Read the model definition and answer for the solid it produces. Units are mm, in the model's axes. Coordinates: 2 decimals unless noted, no trailing zeros. Loops run counter-clockwise (first coordinate to the right, second up) from the corner with the lowest first, then second, coordinate; pieces in that order, holes last. Notation, with made-up numbers: M 67.25,47 L 87.25,47 A10 ccw 87.25,60 Z; hole C 24.25,-1 d11. An arc over 180 degrees is marked long. One line per item, written item: value. Start each with the question number.
1. The part is cut by section B-B (x = 136.5). Write down the section's boundary in (y, z), then the cut area to 3 significant figures.
2. Consider probe 1 along Z at (x, y) = (167, -39.5). Determine where the line is inside the solid, lowest interval first.
3. The part is cut by section A-A (z = -138.5). Write down the section's boundary in (x, y), then the cut area to 3 significant figures.
4. The part is cut by section C-C (y = 100). Write down the section's boundary in (x, z).
5. Flat-ended cylindrical pins translate along their axes: pin 1 (6.5 mm diameter, centred on x = -4, z = -214.5, fed in from -Y); pin 2 (5.5 mm diameter, centred on x = 124.5, z = 2, fed in from -Y); pin 3 (5 mm diameter, centred on x = 287.5, z = -217, fed in from -Y). Find the tip coordinate at first contact, or state that the pin passes through.
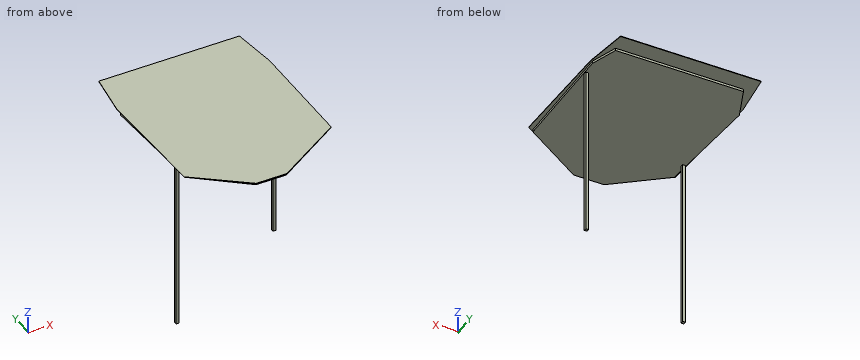
```python
from build123d import *

# Parameters (mm, degrees)
ESQUISSE1_W        = 50
ESQUISSE1_H        = 50
BOSS_EXTRU_1_DEPTH = 5
BOSS_EXTRU_2_DEPTH = 5
ESQUISSE3_W        = 6
ESQUISSE3_H        = 6
BOSS_EXTRU_3_DEPTH = 350
BOSS_EXTRU_4_DEPTH = 1


with BuildPart() as part:
    # Esquisse1 → Boss.-Extru.1 (new body)
    with BuildSketch(Plane.XY):
        with Locations((25, 25)):
            Rectangle(ESQUISSE1_W, ESQUISSE1_H)
    extrude(amount=BOSS_EXTRU_1_DEPTH)

    # Esquisse2 → Boss.-Extru.2 (add)
    with BuildSketch(Plane.XY.offset(5)):
        Polygon((-17.13807747, 66.750016637), (11.246380261, 134.000915956), (274.564409595, 134.000915956), (292.219085418, 78.963245992), (285.658191139, -157.093376415), (157.625700404, -238.014344585), (94.995088054, -238.014344585), (-5.374322013, -157.093376415), align=None)
    extrude(amount=-BOSS_EXTRU_2_DEPTH)

    # Esquisse3 → Boss.-Extru.3 (add)
    with BuildSketch(Plane(origin=(0, 0, 0), x_dir=(-1, 0, 0), z_dir=(0, 0, -1))):
        with Locations((3, -118.721693301)):
            Rectangle(ESQUISSE3_W, ESQUISSE3_H)
        with Locations((-287, 47.238939464)):
            Rectangle(ESQUISSE3_W, ESQUISSE3_H)
    extrude(amount=BOSS_EXTRU_3_DEPTH)

    # Esquisse4 → Boss.-Extru.4 (add)
    with BuildSketch(Plane.XY.offset(5)):
        Polygon((-5.533858716, 170.143499993), (283.889977684, 170.143499993), (295.480369275, 77.420367263), (295.480369275, -154.566750541), (156.395670181, -241.735343219), (93.529944497, -241.735343219), (-10.909112788, -161.778438909), (-18.300087136, 77.420367263), align=None)
    extrude(amount=BOSS_EXTRU_4_DEPTH)


solid = part.part
```
Answer block:
1. outline: M -241.74,5 L -238.01,5 L -238.01,0 L 134,0 L 134,5 L 170.14,5 L 170.14,6 L -241.74,6 Z
1. area: 2,270 mm2
2. probe 1: z = 0 to 6
3. outline: M -6,-121.72 L 0,-121.72 L 0,-115.72 L -6,-115.72 Z; M 284,44.24 L 290,44.24 L 290,50.24 L 284,50.24 Z
3. area: 72.0 mm2
4. outline: M -15.19,5 L -3.1,5 L -3.1,0 L 285.47,0 L 285.47,5 L 292.66,5 L 292.66,6 L -15.19,6 Z
5. pin 1: stops at y = -121.72
5. pin 2: stops at y = -238.01
5. pin 3: stops at y = 44.24
